Autodesk Inventor part; units mm, degrees
ref_plane "YZ Plane" through (0, 0, 0) normal (1, 0, 0) x (0, 1, 0)
ref_plane "XZ Plane" through (0, 0, 0) normal (0, 1, 0) x (-1, 0, 0)
ref_plane "XY Plane" through (0, 0, 0) normal (0, 0, 1) x (1, 0, 0)
sketch "Sketch1" plane through (0, 0, 0) normal (0, 0, 1) x (1, 0, 0)
  line L0 (90.331, -15) -> (-48.669, -15)
  line L1 (-48.669, -15) -> (-48.669, 30)
  line L2 (-48.669, 30) -> (90.331, 30)
  line L3 (90.331, 30) -> (90.331, -15)
  line L4 (3.6008, 15) -> (3.6008, 14)
  line L5 (3.6008, 15) -> (38.0611, 15)
  line L6 (38.0611, 15) -> (38.0611, 14)
  line L7 (38.0611, 14) -> (3.6008, 14)
  arc A0 (1.6411, 15) -> (0, 14) centre (6, 6) ccw
  line L8 (0, 14) -> (34.0626, 14)
  line L9 (34.0626, 15) -> (34.0626, 14)
  line L10 (34.0626, 15) -> (1.6411, 15)
  line L11 (3.6008, 15) -> (-2.0587, 15)
  line L12 (-17.3084, 15) -> (-2.0587, 15)
  line L13 (38.0611, 0) -> (3.6008, 0)
  line L14 (-2.0587, 0) -> (3.6008, 0)
  line L15 (70.331, 14) -> (63.6008, 14)
  arc A1 (70.331, 1) -> (70.331, 14) centre (70.331, 7.5) ccw
  line L16 (63.6008, 1) -> (70.331, 1)
  line L17 (63.6008, 14) -> (63.6008, 1)
  line L18 (-21.9389, 14) -> (-28.669, 14)
  line L19 (-21.9389, 1) -> (-21.9389, 14)
  line L20 (-28.669, 1) -> (-21.9389, 1)
  arc A2 (-28.669, 14) -> (-28.669, 1) centre (-28.669, 7.5) ccw
  arc A3 (-28.669, 15) -> (-28.669, 0) centre (-28.669, 7.5) ccw
  arc A4 (70.331, 0) -> (70.331, 15) centre (70.331, 7.5) ccw
  point P0 (0, 0)
  point P1 (20.831, 30)
  dimension "d0" = 15
  dimension "d1" = 15
  dimension "d2" = 20
  dimension "d3" = 20
extrude "Extrusion1" add sketch "Sketch1" along normal blind 1.5 contours L0 L1 L2 L3 | L5 L9 L7 L4 | L4 L8 A0 L10 | L5 L6 L7 L9 | A1 L16 L17 L15 | L19 L20 A2 L18
sketch "Sketch2" plane through (0, 0, 0) normal (0, 0, -1) x (-1, 0, 0)
  line L0 (-6, 15) -> (-6, 0)
  line L1 (-31.6619, 15) -> (-6, 15)
  line L2 (-31.6619, 0) -> (-31.6619, 15)
  line L3 (-31.6619, 0) -> (-6, 0)
  line L4 (-90.331, 30) -> (48.669, 30)
  line L5 (-90.331, 30) -> (48.669, 30)
  line L6 (-90.331, -15) -> (-90.331, 30)
  line L7 (48.669, -15) -> (-90.331, -15)
  line L8 (48.669, 30) -> (48.669, -15)
  line L9 (-5.8, 15.2) -> (-5.8, -0.2)
  line L10 (-5.8, -0.2) -> (-31.8619, -0.2)
  line L11 (-31.8619, -0.2) -> (-31.8619, 15.2)
  line L12 (-31.8619, 15.2) -> (-5.8, 15.2)
  line L13 (-41.8619, 20.2) -> (5, 20.2)
  line L14 (5, 20.2) -> (5, -5.2)
  line L15 (5, -5.2) -> (-41.8619, -5.2)
  line L16 (-41.8619, -5.2) -> (-41.8619, 20.2)
  line L17 (-34.0626, 1) -> (0, 1)
  line L18 (-34.0626, 14) -> (-34.0626, 1)
  line L19 (0, 14) -> (-34.0626, 14)
  line L20 (0, 1) -> (0, 14)
  point P0 (0, 0)
  point P1 (-31.8619, 1)
  point P2 (-31.8619, 14)
  point P3 (-5.8, 14)
  point P4 (-5.8, 1)
  dimension "d6" = 0.2
  dimension "d7" = 5
  dimension "d8" = 10
  dimension "d9" = 5
  dimension "d10" = 5
extrude "Extrusion2" add sketch "Sketch2" along normal blind 3 contours L13 L14 L15 L16
properties part number "backplate"
Geometry check sheet. Reference: the model listing, model coordinates, mm. A direction names the side the tool comes from. Coordinates: 2 decimals unless noted, no trailing zeros. Order: outer loops, then holes, each group sorted by start corner. A loop starts at its lowest first (then second) coordinate and runs counter-clockwise, first axis right, second up. Notation, with made-up numbers: (32, -20.75) - (66, -20.75) arc R26 ccw to (66, -0.75) - close; hole circle Ø11 at (-35, -21.5). An arc over 180 degrees is marked (long way). Answer in a Markdown table with one row per item. Add a question column.
1. Section check B-B (z = -0.7). Enter the section's corners in (x, y).
2. Section check C-C (x = 36). Enter the section's corners in (y, z).
3. Material ranges on L1, parallel to X at y = 4.5, z = -2.65; L2, parallel to Z at x = -35.5, y = 2.5; L3, parallel to Y at x = -1, z = -1.15, recorded low to high. Write a range as [from, to].
4. Section check D-D (y = 6). Enter the section's corners in (x, z), plus the area to 3 significant figures.
5. Section check A-A (y = 19). Enter the section's corners in (x, z), plus the area to 3 significant figures.
6. Access from +Z, -Z, +X, -X, +Y, -Y to the whole of each face (thin tool, end or side, straight path). Record for faces 5 (the face through (19, -1, -3)), 6 (the face through (-5, 8, -1)), 7 (the face through (34.063, 8, -1)).
7. Draft check along Y on faces 1 (the face through (18, -5.2, -1)), 2 (the face through (19, 20.2, -1)), 3 (the face through (0, 7, -1)), 4 (the face through (41.862, 7, -1)). Enter one of: +Y half, -Y half, draft (parallel to the pull), parting line (faces both ways), or undercut.
8. Gauge pin test, flat ends, axial feed: pin 1 Ø1.3 at (y, z) = (0.5, -1) entering from -X; pin 2 Ø1.5 at (x, z) = (23, -2) entering from -Y; pin 3 Ø2.5 at (y, z) = (10.5, -1.5) entering from +X. Record the tip position at first contact, or that the pin passes through.
Data:
| question | item | result |
|---|---|---|
| 1 | outline | (-5, -5.2) - (41.86, -5.2) - (41.86, 20.2) - (-5, 20.2) - close; hole (0, 1) - (5.8, 1) - (5.8, -0.2) - (31.86, -0.2) - (31.86, 1) - (34.06, 1) - (34.06, 14) - (31.86, 14) - (31.86, 15.2) - (5.8, 15.2) - (5.8, 14) - (0, 14) - close |
| 2 | outline | (-15, 0) - (-5.2, 0) - (-5.2, -3) - (20.2, -3) - (20.2, 0) - (30, 0) - (30, 1.5) - (-15, 1.5) - close |
| 3 | L1 | x = [-5, 0], [34.06, 41.86] |
| 3 | L2 | z = [0, 1.5] |
| 3 | L3 | y = [-5.2, 20.2] |
| 4 | outline | (-48.67, 0) - (-5, 0) - (-5, -3) - (0, -3) - (0, 0) - (34.06, 0) - (34.06, -3) - (41.86, -3) - (41.86, 0) - (90.33, 0) - (90.33, 1.5) - (-48.67, 1.5) - close |
| 4 | area | 247 mm² |
| 5 | outline | (-48.67, 0) - (-5, 0) - (-5, -3) - (41.86, -3) - (41.86, 0) - (90.33, 0) - (90.33, 1.5) - (-48.67, 1.5) - close |
| 5 | area | 349 mm² |
| 6 | face 5 | -Z, +X, -X, +Y, -Y |
| 6 | face 6 | -Z, -X, +Y, -Y |
| 6 | face 7 | -Z |
| 7 | face 1 | -Y half |
| 7 | face 2 | +Y half |
| 7 | face 3 | undercut |
| 7 | face 4 | draft |
| 8 | pin 1 | stops at x = -5 |
| 8 | pin 2 | stops at y = -5.2 |
| 8 | pin 3 | stops at x = 41.86 |
